Could you check a few things on this drawing? It's one solid part, dimensions in mm from its lowest x, y, z. A direction names the side the tool comes from. Round coordinates to 2 decimals unless told otherwise and drop trailing zeros. Write each loop counter-clockwise with the first axis right and the second up, starting at its lowest first coordinate (ties: lowest second). Pieces come first, ordered by that corner, then holes. Notation, with made-up numbers: (88, 58.25) -> (94, 58.25) arc R29 cw to (94, 94.25) -> close; hole circle Ø4 at (-39.5, 63.5). An arc over 180 degrees is marked (long way). Put each result on its own line as item: value. Start each with the question number.
1) I want a section at D-D, the plane x = 11. List the corners of the cut face in (y, z) for me.
2) I want a section at B-B, the plane y = 5. List the corners of the cut face in (x, z) for me (1 decimal).
3) Will these pins go through, and if not, where does the flat tip stop? P1, Ø6, axis at x = 11.5, z = 23, coming from the +Y side; P2, Ø2, axis at x = 6, z = 16.5, coming from the -Y side; P3, Ø4, axis at y = 12.5, z = 16.5, coming from the +X side; P4, Ø1.5, axis at x = 7.5, z = 32.5, coming from the +Y side.
4) I want a section at A-A, the plane y = 15. List the corners of the cut face in (x, z) for me (1 decimal).
5) If I drill on line 1 along Y through (x, z) = (7, 34.75); line 2 along Z through (x, y) = (8.75, 17.5); line 3 along Y through (x, z) = (0.5, 21), over which ranges is the centre line in solid material (lowest first)? Write a range as [from, to].
6) Which directions (+Z, -Z, +X, -X, +Y, -Y) give clear straight access to the entire face, cutting with the end or side of a thin tool? Please do the marked faces 1, 2, 3 and 4.
7) I want a section at C-C, the plane x = 6. List the corners of the cut face in (y, z) for me, then the cut area to 3 significant figures.
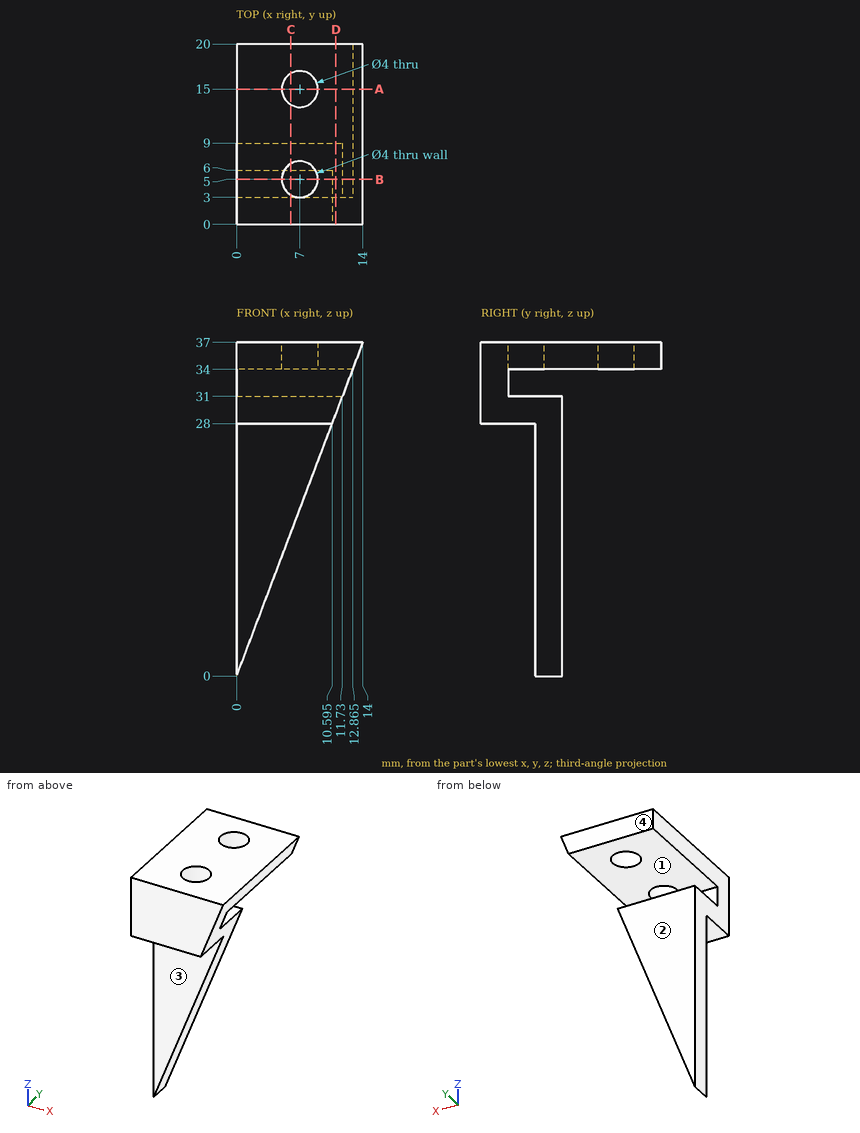
Findings:
1. outline: (0, 29.07) -> (9, 29.07) -> (9, 31) -> (3, 31) -> (3, 34) -> (20, 34) -> (20, 37) -> (0, 37) -> close
2. outline: (0, 28) -> (10.6, 28) -> (11.7, 31) -> (0, 31) -> close; (0, 34) -> (5, 34) -> (5, 37) -> (0, 37) -> close; (9, 34) -> (12.9, 34) -> (14, 37) -> (9, 37) -> close
3. P1: stops at y = 9
3. P2: stops at y = 6
3. P3: passes through
3. P4: stops at y = 3
4. outline: (0, 34) -> (5, 34) -> (5, 37) -> (0, 37) -> close; (9, 34) -> (12.9, 34) -> (14, 37) -> (9, 37) -> close
5. line 1: y = [0, 3], [7, 13], [17, 20]
5. line 2: z = [34, 37]
5. line 3: y = [6, 9]
6. face 1: +X, -X, +Y
6. face 2: -Z, +X, -X, +Y
6. face 3: -Z, +X, -X, -Y
6. face 4: +Z, -Z, +X, -X, +Y
7. outline: (0, 28) -> (6, 28) -> (6, 15.86) -> (9, 15.86) -> (9, 31) -> (3, 31) -> (3, 34) -> (3.27, 34) -> (3.27, 37) -> (0, 37) -> close; (6.73, 34) -> (13.27, 34) -> (13.27, 37) -> (6.73, 37) -> close; (16.73, 34) -> (20, 34) -> (20, 37) -> (16.73, 37) -> close
7. area: 112 mm2
